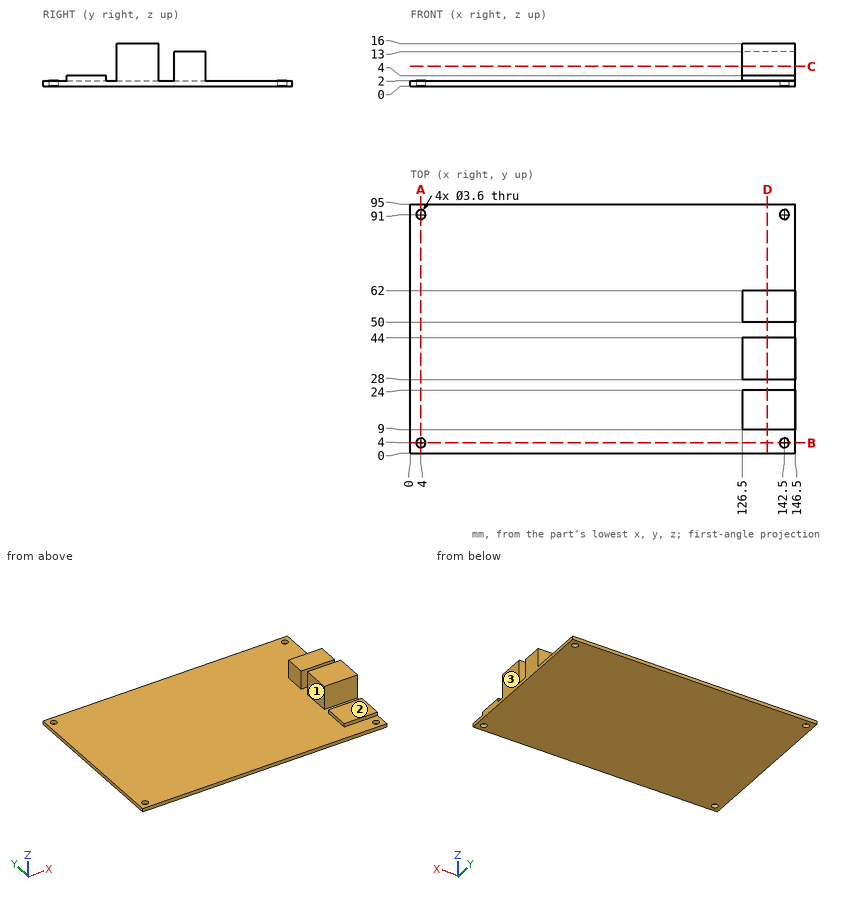
The figure shows three views and two pictorial views of one solid part (mm, origin at its lowest corner). Answer the questions. A direction names the side the tool comes from. Coordinates: 2 decimals unless noted, no trailing zeros. Order: outer loops, then holes, each group sorted by start corner. A loop starts at its lowest first (then second) coordinate and runs counter-clockwise, first axis right, second up.
Q1. Given P1, Ø9, axis at x = 140.5, z = 7, coming from the +Y side; P2, Ø6, axis at x = 142.5, y = 91, coming from the +Z side; P3, Ø1.6, axis at x = 139.5, z = 3, coming from the -Y side, each flat-ended and moving along its own axis, determine where each tip first touches the part or whether it passes through.
Q2. A cutting plane is placed at C-C, the plane z = 7.5. Write down the section's boundary in (x, y).
Q3. A cutting plane is placed at D-D, the plane x = 136. Write down the section's boundary in (y, z), and give its area (3 significant figures).
Q4. A cutting plane is placed at A-A, the plane x = 4. Write down the section's boundary in (y, z).
Q5. Which of the six approach directions +Z, -Z, +X, -X, +Y, -Y give full straight-line access (tool end or side, diameter ignored) to the marked faces 1, 2 and 3?
Q6. Consider line 1 (X direction, y = 91, z = 1.5); line 2 (Y direction, x = 142.5, z = 1.55); line 3 (Z direction, x = 113, y = 40.5). Determine where each line is inside the solid, lowest interval first.
Q7. A cutting plane is placed at B-B, the plane y = 4. Write down the section's boundary in (x, z), and give its area (3 significant figures).
Answers follow:
1. P1: stops at y = 62
1. P2: stops at z = 2
1. P3: stops at y = 9
2. outline: (126.5, 28) - (146.5, 28) - (146.5, 44) - (126.5, 44) - close; (126.5, 50) - (146.5, 50) - (146.5, 62) - (126.5, 62) - close
3. outline: (0, 0) - (95, 0) - (95, 2) - (62, 2) - (62, 13) - (50, 13) - (50, 2) - (44, 2) - (44, 16) - (28, 16) - (28, 2) - (24, 2) - (24, 4) - (9, 4) - (9, 2) - (0, 2) - close
3. area: 576 mm2
4. outline: (0, 0) - (2.2, 0) - (2.2, 2) - (0, 2) - close; (5.8, 0) - (89.2, 0) - (89.2, 2) - (5.8, 2) - close; (92.8, 0) - (95, 0) - (95, 2) - (92.8, 2) - close
5. face 1: +Z, -X, +Y, -Y
5. face 2: +Z, +X, -X, -Y
5. face 3: +Z, -Z, +X, +Y, -Y
6. line 1: x = 0 to 2.2, 5.8 to 140.7, 144.3 to 146.5
6. line 2: y = 0 to 2.2, 5.8 to 89.2, 92.8 to 95
6. line 3: z = 0 to 2
7. outline: (0, 0) - (2.2, 0) - (2.2, 2) - (0, 2) - close; (5.8, 0) - (140.7, 0) - (140.7, 2) - (5.8, 2) - close; (144.3, 0) - (146.5, 0) - (146.5, 2) - (144.3, 2) - close
7. area: 279 mm2
